```python
from build123d import *

# Parameters (mm, degrees)
SKETCH1_R           = 1.6
SKETCH1_R_2         = 1.05
BOSS_EXTRUDE1_DEPTH = 7
SKETCH2_R           = 2
CUT_EXTRUDE1_DEPTH  = 2


with BuildPart() as part:
    # Sketch1 → Boss-Extrude1 (new body)
    with BuildSketch(Plane.XY):
        with BuildLine():
            Line((0, 0), (17, 0))
            ThreePointArc((17, 0), (19.121320344, 0.878679656), (20, 3))
            Line((20, 3), (20, 17))
            ThreePointArc((20, 17), (19.121320344, 19.121320344), (17, 20))
            Line((17, 20), (0, 20))
            Line((0, 20), (0, 0))
        make_face()
        with Locations((5.2, 16)):
            Circle(SKETCH1_R, mode=Mode.SUBTRACT)
        with Locations((14.8, 16)):
            Circle(SKETCH1_R, mode=Mode.SUBTRACT)
        with Locations((5.2, 6.5)):
            Circle(SKETCH1_R_2, mode=Mode.SUBTRACT)
        with Locations((14.8, 6.5)):
            Circle(SKETCH1_R_2, mode=Mode.SUBTRACT)
    extrude(amount=BOSS_EXTRUDE1_DEPTH)

    # Sketch2 → Cut-Extrude1 (cut)
    with BuildSketch(Plane.XY.offset(7)):
        with Locations((5.2, 6.5)):
            Circle(SKETCH2_R)
        with Locations((14.8, 6.5)):
            Circle(SKETCH2_R)
    extrude(amount=-CUT_EXTRUDE1_DEPTH, mode=Mode.SUBTRACT)


solid = part.part
```
For this review, take the finished solid that the model builds, in its own axes (mm). A direction names the side the tool comes from. Round coordinates to 2 decimals unless told otherwise and drop trailing zeros. Write each loop counter-clockwise with the first axis right and the second up, starting at its lowest first coordinate (ties: lowest second). Pieces come first, ordered by that corner, then holes.
1) For line 1 along X through (y, z) = (6.5, 2.9); line 2 along Y through (x, z) = (14.8, 3.1); line 3 along Y through (x, z) = (14, 5.25), list the stretches that pass through material, from the lowest coordinate up.
Answer below:
line 1: x = 0 to 4.15, 6.25 to 13.75, 15.85 to 20
line 2: y = 0 to 5.45, 7.55 to 14.4, 17.6 to 20
line 3: y = 0 to 4.67, 8.33 to 14.61, 17.39 to 20
2) Take a section at A-A on x = 14.8. Give the boundary of the cut face in (y, z).
Answer below:
outline: (0, 0) - (5.45, 0) - (5.45, 5) - (4.5, 5) - (4.5, 7) - (0, 7) - close; (7.55, 0) - (14.4, 0) - (14.4, 7) - (8.5, 7) - (8.5, 5) - (7.55, 5) - close; (17.6, 0) - (20, 0) - (20, 7) - (17.6, 7) - close
3) Insertion check: pin 1 Ø3.5 at (x, y) = (5.2, 6.5) entering from +Z. The pin has a flat end and moves straight along its axis. Give the tip position at first contact, or say it passes through.
Answer below:
pin 1: stops at z = 5
4) Take a section at B-B on z = 2. Give the boundary of the cut face in (x, y), then the cut area to 3 significant figures.
Answer below:
outline: (0, 0) - (17, 0) arc R3 ccw to (20, 3) - (20, 17) arc R3 ccw to (17, 20) - (0, 20) - close; hole circle Ø3.2 at (5.2, 16); hole circle Ø2.1 at (5.2, 6.5); hole circle Ø3.2 at (14.8, 16); hole circle Ø2.1 at (14.8, 6.5)
area: 373 mm2
5) Machinability: for faces 1 (the face through (12.802, 6.588, 6.014)), 2 (the face through (10, 10, 0)), which of the approach directions +Z, -Z, +X, -X, +Y, -Y give a long, thin tool a straight path to every point of the face, cutting with its end or side? Answer none if there is none.
Answer below:
face 1: +Z
face 2: -Z, +X, -X, +Y, -Y
6) Take a section at C-C on y = 6.5. Give the boundary of the cut face in (x, z), then the cut area to 3 significant figures.
Answer below:
outline: (0, 0) - (4.15, 0) - (4.15, 5) - (3.2, 5) - (3.2, 7) - (0, 7) - close; (6.25, 0) - (13.75, 0) - (13.75, 5) - (12.8, 5) - (12.8, 7) - (7.2, 7) - (7.2, 5) - (6.25, 5) - close; (15.85, 0) - (20, 0) - (20, 7) - (16.8, 7) - (16.8, 5) - (15.85, 5) - close
area: 103 mm2
7) Mouldability with a two-part tool opening along Y and no side actions: class faces 3 (the face through (9, 20, 3)), 4 (the face through (20, 10, 3)), 5 (the face through (6.1, 5.6, 5)) as +Y half, -Y half, draft (parallel to the pull), parting line (faces both ways), or undercut.
Answer below:
face 3: +Y half
face 4: draft
face 5: undercut
8) Take a section at D-D on y = 16.5. Give the boundary of the cut face in (x, z), then the cut area to 3 significant figures.
Answer below:
outline: (0, 0) - (3.68, 0) - (3.68, 7) - (0, 7) - close; (6.72, 0) - (13.28, 0) - (13.28, 7) - (6.72, 7) - close; (16.32, 0) - (20, 0) - (20, 7) - (16.32, 7) - close
area: 97.4 mm2
